Read the model definition and answer for the solid it produces. Units are mm, in the model's axes. Face numbers are marked on the shaded views. A direction names the side the tool comes from. Round coordinates to 2 decimals unless told otherwise and drop trailing zeros. Write each loop counter-clockwise with the first axis right and the second up, starting at its lowest first coordinate (ties: lowest second). Pieces come first, ordered by that corner, then holes. Notation, with made-up numbers: (36, 6.5) -> (88, 6.5) arc R23 ccw to (88, 19.5) -> close; hole circle Ø10 at (-14.5, -30.5). An arc over 180 degrees is marked (long way). Return JSON: item names as keys, results as strings. Group by question number.
(1) For the marked faces 4, 5, 6 and 7, determine the directions among +Z, -Z, +X, -X, +Y, -Y from which every point of the face is accessible in a straight line to the end or side of a thin tool.
(2) A cutting plane is placed at D-D on y = 42.5. Give the vertices of the cut face in (x, z).
(3) Straight lines are drawn through the part: line 1 (Y direction, x = -1.5, z = 0) (3 decimals); line 2 (Y direction, x = 3.5, z = 2) (3 decimals); line 3 (X direction, y = 48, z = -0.25). For each, find the intervals that lie inside material, in ascending order.
(4) A cutting plane is placed at A-A on z = 0. Give the vertices of the cut face in (x, y) (3 decimals), then the cut area to 3 significant figures.
(5) A cutting plane is placed at B-B on y = 6.35. Give the vertices of the cut face in (x, z) (3 decimals).
(6) Given pin 1 (6 mm diameter, centred on y = 23, z = -1.5, fed in from +X); pin 2 (3 mm diameter, centred on y = 11, z = 4.5, fed in from +X) (3 decimals); pin 3 (7.5 mm diameter, centred on y = 7, z = 0.5, fed in from -X) (3 decimals), each flat-ended and moving along its own axis, determine where each tip first touches the part or whether it passes through.
(7) The mould has two halves that part along Y. Classify the marked faces 1, 2 and 3: released by +Y, released by -Y, zero draft, split by the parting line, or undercut.
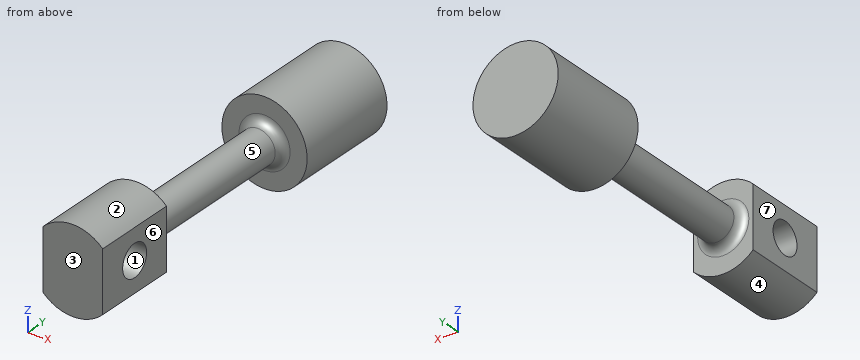
```python
from build123d import *

# Parameters (mm, degrees)
SKETCH1_R                      = 6.35
BOSS_EXTRUDE1_DEPTH            = 53.975
SKETCH3_W                      = 13.824388351
SKETCH3_H                      = 22.988870516
CUT_EXTRUDE1_DEPTH             = 55.716959208
F_3_16_0_1875_DIAMETER_HOLE1_D = 4.7625


with BuildPart() as part:
    # Sketch1 → Boss-Extrude1 (new body)
    with BuildSketch(Plane(origin=(0, 0, 0), x_dir=(1, 0, 0), z_dir=(0, 1, 0))):
        with Locations(Location((0, 0, 0), (0, 0, 270))):
            Circle(SKETCH1_R)
    extrude(amount=BOSS_EXTRUDE1_DEPTH)

    # Sketch2 → Cut-Revolve1 (revolve, cut)
    with BuildSketch(Plane.XY, mode=Mode.PRIVATE) as cut_revolve1_sk:
        with BuildLine():
            Line((26.057124612, 38.1), (3.81, 38.1))
            ThreePointArc((3.81, 38.1), (2.911974388, 37.728025612), (2.54, 36.83))
            Line((2.54, 36.83), (2.54, 13.97))
            ThreePointArc((2.54, 13.97), (2.911974388, 13.071974388), (3.81, 12.7))
            Line((3.81, 12.7), (26.057124612, 12.7))
            Line((26.057124612, 12.7), (26.057124612, 38.1))
        make_face()
    revolve(cut_revolve1_sk.sketch.rotate(Axis((0, 0, 0), (0, 1, 0)), 90), axis=Axis((0, 0, 0), (0, 1, 0)), mode=Mode.SUBTRACT)

    # Sketch3 → Cut-Extrude1 (cut, symmetric)
    with BuildSketch(Plane.XY):
        with Locations((11.357194176, 7.862043189)):
            Rectangle(SKETCH3_W, SKETCH3_H)
    cut_extrude1 = extrude(amount=CUT_EXTRUDE1_DEPTH, both=True, mode=Mode.SUBTRACT)

    # Mirror1: Cut-Extrude1 across plane
    add(cut_extrude1.mirror(Plane(origin=(0, 0, 0), x_dir=(0, 0, 1), z_dir=(1, 0, 0))), mode=Mode.SUBTRACT)

    # 3/16 (0.1875) Diameter Hole1 (through all)
    with Locations(Plane.ZY.offset(4.445)):
        with Locations((0, 6.35)):
            Hole(F_3_16_0_1875_DIAMETER_HOLE1_D / 2)


solid = part.part
```
Checks:
{
 "1": {"face 4": "-Z, +Y, -Y", "face 5": "none", "face 6": "+Z, -Z, +X, -Y", "face 7": "+Z, -Z, -X, -Y"},
 "2": {"outline": "circle Ø12.7 at (0, 0)"},
 "3": {"line 1": "y = 0 to 3.969, 8.731 to 53.975", "line 2": "y = 0 to 5.058, 7.642 to 12.7, 38.1 to 53.975", "line 3": "x = -6.35 to 6.35"},
 "4": {"outline": "(-6.35, 38.1) -> (-3.81, 38.1) arc R1.27 cw to (-2.54, 36.83) -> (-2.54, 13.97) arc R1.27 cw to (-3.81, 12.7) -> (-4.445, 12.7) -> (-4.445, 8.731) -> (4.445, 8.731) -> (4.445, 12.7) -> (3.81, 12.7) arc R1.27 cw to (2.54, 13.97) -> (2.54, 36.83) arc R1.27 cw to (3.81, 38.1) -> (6.35, 38.1) -> (6.35, 53.975) -> (-6.35, 53.975) -> close; (-4.445, 0) -> (4.445, 0) -> (4.445, 3.969) -> (-4.445, 3.969) -> close", "area": "403 mm^2"},
 "5": {"outline": "(-4.445, -4.535) arc R6.35 ccw to (4.445, -4.535) -> (4.445, -2.381) -> (-4.445, -2.381) -> close; (-4.445, 2.381) -> (4.445, 2.381) -> (4.445, 4.535) arc R6.35 ccw to (-4.445, 4.535) -> close"},
 "6": {"pin 1": "stops at x = 2.54", "pin 2": "stops at x = 4.445", "pin 3": "stops at x = -4.445"},
 "7": {"face 1": "undercut", "face 2": "zero draft", "face 3": "released by -Y"}
}
